Solid Edge part; units mm, degrees
sketch "Sketch1" plane through (0, 0, 0) normal (0, 1, 0) x (-1, 0, 0)
  circle A0 centre (0, 0) radius 17.5
  circle A1 centre (0, 0) radius 39
extrude "Protrusion1" add sketch "Sketch1" against normal blind 10
sketch "Sketch2" plane through (0, 0, 0) normal (0, 1, 0) x (0, 0, 1)
  circle A0 centre (-20.8226, 21.5968) radius 2.25
  circle A1 centre (17.6529, 24.2565) radius 2.25
  circle A2 centre (29.1146, 7.2345) radius 2.25
  circle A3 centre (26.9533, -13.1726) radius 2.25
  circle A4 centre (12.1803, -27.4161) radius 2.25
  circle A5 centre (-8.2921, -28.8313) radius 2.25
  circle A6 centre (-24.8845, -16.756) radius 2.25
extrude "ExtrudedCutout_1" cut sketch "Sketch2" against normal blind 130.6
sketch "Sketch3" plane through (0, 0, 0) normal (0, 1, 0) x (-1, 0, 0)
  circle A0 centre (0, 32) radius 2.8
  circle A1 centre (-32, 0) radius 2.8
  circle A2 centre (0, -32) radius 2.8
  circle A3 centre (32, 0) radius 2.8
extrude "ExtrudedCutout_2" cut sketch "Sketch3" against normal blind 261.7
sketch "Sketch4" plane through (0, -10, 0) normal (0, -1, 0) x (0, 0, 1)
  circle A0 centre (0, 32) radius 2.8
  line L0 (0, 36.5) -> (-3.8971, 34.25)
  line L1 (-3.8971, 34.25) -> (-3.8971, 29.75)
  line L2 (-3.8971, 29.75) -> (0, 27.5)
  line L3 (0, 27.5) -> (3.8971, 29.75)
  line L4 (3.8971, 29.75) -> (3.8971, 34.25)
  line L5 (3.8971, 34.25) -> (0, 36.5)
extrude "ExtrudedCutout_3" cut sketch "Sketch4" against normal blind 4
pattern_circular "Pattern1" count 4 over 360 about axis through (0, -10, 0) along (0, -1, 0) of "ExtrudedCutout_3"
sketch "Sketch5" plane through (0, 0, 0) normal (0, 1, 0) x (1, 0, 0)
  circle A0 centre (-16.756, 24.8845) radius 4
  circle A1 centre (21.5968, 20.8226) radius 4
  circle A2 centre (24.2565, -17.6529) radius 4
  circle A3 centre (7.2345, -29.1146) radius 4
  circle A4 centre (-13.1726, -26.9533) radius 4
  circle A5 centre (-27.4161, -12.1803) radius 4
  circle A6 centre (-28.8313, 8.2921) radius 4
extrude "ExtrudedCutout_4" cut sketch "Sketch5" against normal blind 3
Geometry check sheet. Reference: the model listing, model coordinates, mm. A direction names the side the tool comes from. Give positions to 0.01 mm unless a question says otherwise; leave off trailing zeros. Loops run counter-clockwise (first coordinate to the right, second up) from the corner with the lowest first, then second, coordinate; pieces in that order, holes last. Notation, with made-up numbers: M 70.25,-6 L 78.25,-6 A23 ccw 78.25,16 Z; hole C 35.25,39.5 d6. An arc over 180 degrees is marked long. Answer as CSV lines item,"result".
Item 1: Cross-section at B-B on y = -7.75. Count the separate pieces of the cut face and the enclosed holes in it, and give its area (3 significant figures).
Values:
separate pieces,"1"
enclosed holes,"12"
area,"3,490 mm²"
Item 2: Release check for a two-part mould opening along X. For faces 4 (the cylindrical face through (5.077, -4.93, 38.668)), 5 (the flat face through (-1.92, -8.03, -28.61)) record: pulls with the +X half, pulls with the -X half, needs draft (parallel to the pull), parting line crosses it, or undercut.
Values:
face 4,"parting line crosses it"
face 5,"undercut"
Item 3: Cross-section at C-C on x = 32. Record the cut outline in (y, z), and give its area (3 significant figures).
Values:
outline,"M -10,-22.29 L 0,-22.29 L 0,-2.8 L -6,-2.8 L -6,-3.9 L -10,-3.9 Z; M -10,3.9 L -6,3.9 L -6,2.8 L 0,2.8 L 0,22.29 L -10,22.29 Z"
area,"381 mm²"
Item 4: Cross-section at A-A on z = -32. Record the cut outline in (x, y), and give its area (3 significant figures).
Values:
outline,"M -22.29,-10 L -3.9,-10 L -3.9,-6 L -2.8,-6 L -2.8,0 L -22.29,0 Z; M 2.8,-6 L 3.9,-6 L 3.9,-10 L 22.29,-10 L 22.29,0 L 2.8,0 Z"
area,"381 mm²"
Item 5: Access from +Z, -Z, +X, -X, +Y, -Y to the whole of each face (thin tool, end or side, straight path). Record for faces 1 (the cylindrical face through (5.865, -6.451, 27.329)), 2 (the flat face through (35.39, -8.03, 1.92)), 3 (the flat face through (5.5, -3, 30.8)).
Values:
face 1,"+Y, -Y"
face 2,"-Y"
face 3,"+Y"
Item 6: Cross-section at D-D on z = 5. Record the cut outline in (x, y), and give its area (3 significant figures).
Values:
outline,"M -38.68,-10 L -16.77,-10 L -16.77,0 L -38.68,0 Z; M 16.77,-10 L 38.68,-10 L 38.68,0 L 16.77,0 Z"
area,"438 mm²"
Item 7: Depth check by flat-ended pin: P1, Ø3, axis at y = -3, z = -15, coming from the +X side; P2, Ø4, axis at x = -6.5, y = -6.5, coming from the +Z side; P3, Ø8.5, axis at x = -31, z = 1.5, coming from the -Y side; P4, Ø1, axis at y = -8, z = 1.5, coming from the +X side. Enter the tip coordinate at first touch or a pass-through.
Values:
P1,"stops at x = 36.59"
P2,"stops at z = 38.74"
P3,"stops at y = -10"
P4,"stops at x = 38.99"
Item 8: Material ranges on line 1 (X direction, y = -1.5, z = 32); line 2 (X direction, y = -7.5, z = 14); line 3 (Z direction, x = 8, y = -9.5), recorded low to high.
Values:
line 1,"x = -22.29 to -2.8, 2.8 to 4.46, 10 to 22.29"
line 2,"x = -36.4 to -28.74, -26.09 to -10.5, 10.5 to 36.4"
line 3,"z = -38.17 to -15.56, 15.56 to 27, 31.23 to 38.17"
